Input: part model. Units: mm. Frame: model coordinates. A direction names the side the tool comes from. Give positions to 0.01 mm unless a question says otherwise; leave off trailing zeros. Loops run counter-clockwise (first coordinate to the right, second up) from the corner with the lowest first, then second, coordinate; pieces in that order, holes last. Notation, with made-up numbers: (18.5, -3) -> (54.5, -3) arc R32 ccw to (54.5, 32) -> close; hole circle Ø7 at (80, 23). An arc over 180 degrees is marked (long way). Answer as a JSON object with one key per item and string values. Group by question number.
```python
from build123d import *
from build123d.topology import SkipClean

# Parameters (mm, degrees)
SKETCH2_OUTSIDE_W       = 157.722
SKETCH2_OUTSIDE_H       = 157.722
SKETCH2_OUTSIDE_W_2     = 115
SKETCH2_OUTSIDE_H_2     = 40
CUT_EXTRUDE1_DEPTH      = 148.033159525
CUT_EXTRUDE2_DEPTH      = 137.793640203
CUT_EXTRUDE2_DEPTH_BACK = 137.793640203
SKETCH1_4_R             = 37.5
FILLET1_R               = 4
SKETCH3_W               = 1.5
SKETCH3_H               = 2.65
BOSS_EXTRUDE1_START     = 5
BOSS_EXTRUDE1_DEPTH     = 5
CHAMFER1_SIZE           = 0.5


with BuildPart() as part:
    # Sketch1 one side → Revolve1 (revolve)
    with BuildSketch(Plane(origin=(0, 0, 0), x_dir=(1, 0, 0), z_dir=(0, 1, 0))):
        with BuildLine():
            Line((0, 27.5), (0, 102.5))
            ThreePointArc((0, 102.5), (-37.5, 65), (0, 27.5))
        make_face()
        with BuildLine():
            ThreePointArc((37.5, 65), (26.516504294, 91.516504294), (0, 102.5))
            Line((0, 102.5), (0, 27.5))
            ThreePointArc((0, 27.5), (26.516504294, 38.483495706), (37.5, 65))
        make_face()
        with BuildLine():
            ThreePointArc((0, 122.5), (40.658639918, 105.658639918), (57.5, 65))
            Line((57.5, 65), (57.5, 0))
            Line((57.5, 0), (0, 0))
            Line((0, 0), (0, 122.5))
        make_face()
    revolve(axis=Axis((0, 0, 0), (0, 0, -1)))

    # Sketch2 outside → Cut-Extrude1 (cut, through all)
    with BuildSketch(Plane.XY):
        Rectangle(SKETCH2_OUTSIDE_W, SKETCH2_OUTSIDE_H)
        Rectangle(SKETCH2_OUTSIDE_W_2, SKETCH2_OUTSIDE_H_2, mode=Mode.SUBTRACT)
    extrude(amount=-CUT_EXTRUDE1_DEPTH, mode=Mode.SUBTRACT)

    # Sketch1_4 → Cut-Extrude2 (cut, two sides: drawn at the far end of the back side and taken through both)
    with BuildSketch(Plane(origin=(0, 0, 0), x_dir=(1, 0, 0), z_dir=(0, 1, 0)).offset(-CUT_EXTRUDE2_DEPTH_BACK)):
        with Locations(Location((0, 65, 0), (0, 0, 270))):
            Circle(SKETCH1_4_R)
    extrude(amount=CUT_EXTRUDE2_DEPTH + CUT_EXTRUDE2_DEPTH_BACK, mode=Mode.SUBTRACT)

    # Fillet1
    fillet1_edges = [part.edges().sort_by_distance(p)[0] for p in [
        (0, -20, -118.909646632),
        (0, 20, -118.909646632),
        (-53.909646632, 20, -32.5),
        (53.909646632, 20, -32.5),
        (53.909646632, -20, -32.5),
        (-53.909646632, -20, -32.5),
    ]]
    fillet(fillet1_edges, radius=FILLET1_R)

    # Sketch3 → Cut-Revolve1 (revolve, cut)
    with BuildSketch(Plane(origin=(0, 0, 0), x_dir=(0, 0, -1), z_dir=(1, 0, 0))):
        with Locations((103.25, 15.325)):
            Rectangle(SKETCH3_W, SKETCH3_H)
        with Locations((103.25, -15.325)):
            Rectangle(SKETCH3_W, SKETCH3_H)
    revolve(axis=Axis((0, -20, -65), (0, 1, 0)), mode=Mode.SUBTRACT)

    # Sketch4 → Boss-Extrude1 (add)
    with SkipClean():  # the faces are left unmerged after this step: merging them gives an invalid solid
        with BuildSketch(Plane.XY.offset(BOSS_EXTRUDE1_START)):
            with BuildLine():
                Line((-57.445626465, -2.5), (57.445626465, -2.5))
                ThreePointArc((57.445626465, -2.5), (57.486405007, -1.250295697), (57.5, -1.68e-07))
                ThreePointArc((57.5, -1.68e-07), (57.486405011, 1.250295529), (57.445626465, 2.5))
                Line((57.445626465, 2.5), (-57.445626465, 2.5))
                ThreePointArc((-57.445626465, 2.5), (-57.486405007, 1.250295697), (-57.5, 1.68e-07))
                ThreePointArc((-57.5, 1.68e-07), (-57.486405011, -1.250295529), (-57.445626465, -2.5))
            make_face()
        extrude(amount=-BOSS_EXTRUDE1_DEPTH)

    # Chamfer1
    chamfer1_edges = [part.edges().sort_by_distance(p)[0] for p in [
        (0, -20, -102.5),
        (0, 20, -102.5),
        (0, -2.5, 5),
        (0, 2.5, 5),
    ]]
    chamfer(chamfer1_edges, length=CHAMFER1_SIZE)


solid = part.part
```
Q1. Pin query (flat end, axial travel): pin 1 Ø10 at (y, z) = (-12.5, -55.5) entering from -X; pin 2 Ø3 at (y, z) = (2.5, -12.5) entering from +X; pin 3 Ø19 at (x, y) = (-1, 15) entering from +Z; pin 4 Ø6 at (x, z) = (25, -85) entering from +Y. Return the tip coordinate at first contact, or that it passes through.
Q2. Section A-A on z = -17.5. Return the cut outline in (x, y), then the cut area to 3 significant figures.
Q3. Ray query, probe 1 along X at (y, z) = (1.5, -65); probe 2 along Y at (x, z) = (7, -27); probe 3 along Z at (x, y) = (-23.5, -4.5). Return the intervals inside material, ascending.
Q4. Set-up query: faces 1 (the face through (53.45, -19.2, -32.04)), 2 (the face through (1, 2.5, 2)), 3 (the face through (-26.358, 15.344, -36.255)). Return all of +Z, -Z, +X, -X, +Y, -Y with unobstructed straight access to the full face (end or side cutting, diameter ignored); none if empty.
Q5. Pull-direction query (Z, two-part tool) for faces 4 (the face through (-1, -2.5, 2)), 5 (the face through (11.26, -0.2, -29.23)), 6 (the face through (-1, -11, 0)); classes: +Z half, -Z half, draft (parallel to the pull), parting line (faces both ways), or undercut.
Q6. Section B-B on y = 6.5. Return the cut outline in (x, z).
Q7. Section C-C on y = -12. Return the cut outline in (x, z).
Numbers:
{
 "1": {"pin 1": "stops at x = -57.01", "pin 2": "stops at x = 57.49", "pin 3": "stops at z = 0", "pin 4": "passes through"},
 "2": {"outline": "(-54.87, -17.2) arc R4 ccw to (-51.05, -20) -> (51.05, -20) arc R4 ccw to (54.87, -17.2) arc R57.5 ccw to (54.87, 17.2) arc R4 ccw to (51.05, 20) -> (-51.05, 20) arc R4 ccw to (-54.87, 17.2) arc R57.5 ccw to start", "area": "4,500 mm²"},
 "3": {"probe 1": "x = -57.48 to -37.5, 37.5 to 57.48", "probe 2": "y = -20 to -16.65, -14 to 14, 16.65 to 20", "probe 3": "z = -117.29 to -94.22, -35.78 to 0"},
 "4": {"face 1": "+Z, -Z, +X, -Y", "face 2": "+Z, +X, -X, +Y", "face 3": "none"},
 "5": {"face 4": "draft", "face 5": "undercut", "face 6": "+Z half"},
 "6": {"outline": "(-57.13, -65) arc R57.13 ccw to (57.13, -65) -> (57.13, 0) -> (-57.13, 0) -> close; hole circle Ø75 at (0, -65)"},
 "7": {"outline": "(-56.23, -65) arc R56.23 ccw to (56.23, -65) -> (56.23, 0) -> (-56.23, 0) -> close; hole circle Ø75 at (0, -65)"}
}
